For this review, take the finished solid that the model builds, in its own axes (mm). Give positions to 0.01 mm unless a question says otherwise; leave off trailing zeros. Order: outer loops, then holes, each group sorted by start corner. A loop starts at its lowest first (then second) coordinate and runs counter-clockwise, first axis right, second up. Notation, with made-up numbers: (-16, 60.25) -> (26, 60.25) arc R16 cw to (26, 65.25) -> close; hole circle Ø5 at (-20.75, 37). An arc over 180 degrees is marked (long way). Return JSON: item names as keys, results as strings. Group by question number.
1) Add section C-C (z = 1.95). State how many separate pieces and enclosed holes the cut face has, then the cut area to 3 significant figures.
2) Insertion check: P1, Ø3.5, axis at x = 33.61, y = -5.29, coming from the +Z side; P2, Ø1, axis at x = 5, z = 2, coming from the -Y side. Each pin has a flat end and moves straight along its axis. Give the tip position at first contact, or say it passes through.
3) To check wall thickness, follow line 1 along Y through (x, z) = (13, 2.7); line 2 along Y through (x, z) = (3, 1.8); line 3 along Y through (x, z) = (35.5, 1.9). State the ranges of each line that lie inside material, in increasing order.
4) Add section B-B (x = 33). Give the boundary of the cut face in (y, z).
5) Add section D-D (y = 0). Give the boundary of the cut face in (x, z), then the cut area to 3 significant figures.
6) The part is to be moulded in two halves that separate along Y. For faces 1 (the face through (35.094, 10.903, 1.479)), 2 (the face through (-11.237, -34.76, 1.479)), 3 (the face through (-22.86, -10.54, 1.48)), 4 (the face through (19.305, 12.095, 1.479)), say which applies: released by +Y, released by -Y, zero draft, split by the parting line, or undercut.
7) Add section A-A (y = -32). Give the boundary of the cut face in (x, z), then the cut area to 3 significant figures.
from build123d import *

# Parameters (mm, degrees)
SKETCH8_R           = 2.75
SKETCH8_R_2         = 5.3467
BOSS_EXTRUDE1_DEPTH = 3


with BuildPart() as part:
    # Sketch8 → Boss-Extrude1 (new body)
    with BuildSketch(Plane.XY):
        with BuildLine():
            Line((-22.998435926, -22.998435926), (0.859030886, -46.855902739))
            Line((0.859030886, -46.855902739), (46.855902739, -0.859030886))
            Line((46.855902739, -0.859030886), (22.998435926, 22.998435926))
            ThreePointArc((22.998435926, 22.998435926), (10.677524528, 22.998435926), (10.677524528, 10.677524528))
            Line((10.677524528, 10.677524528), (10.668544272, 10.668544272))
            ThreePointArc((10.668544272, 10.668544272), (10.668544272, -10.668544272), (-10.668544272, -10.668544272))
            Line((-10.668544272, -10.668544272), (-10.677524528, -10.677524528))
            ThreePointArc((-10.677524528, -10.677524528), (-22.998435926, -10.677524528), (-22.998435926, -22.998435926))
        make_face()
        with Locations((33.610182952, -5.29098063)):
            Circle(SKETCH8_R, mode=Mode.SUBTRACT)
        with Locations((16.837980227, 16.837980227)):
            Circle(SKETCH8_R_2, mode=Mode.SUBTRACT)
        with Locations((-16.837980227, -16.837980227)):
            Circle(SKETCH8_R_2, mode=Mode.SUBTRACT)
        with Locations((5.325911705, -33.575251877)):
            Circle(SKETCH8_R, mode=Mode.SUBTRACT)
    extrude(amount=BOSS_EXTRUDE1_DEPTH)


solid = part.part
Evaluation:
{
 "1": {"separate pieces": "1", "enclosed holes": "4", "area": "1,850 mm^2"},
 "2": {"P1": "through", "P2": "y = -43.21"},
 "3": {"line 1": "-34.71 to -7.66, 7.66 to 13.12, 20.56 to 24.66", "line 2": "-44.71 to -35.04, -32.11 to -14.79", "line 3": "-12.21 to -7.29, -3.29 to 10.5"},
 "4": {"outline": "(-14.71, 0) -> (-7.97, 0) -> (-7.97, 3) -> (-14.71, 3) -> close; (-2.61, 0) -> (13, 0) -> (13, 3) -> (-2.61, 3) -> close"},
 "5": {"outline": "(15.09, 0) -> (46, 0) -> (46, 3) -> (15.09, 3) -> close", "area": "92.7 mm^2"},
 "6": {"face 1": "released by +Y", "face 2": "released by -Y", "face 3": "split by the parting line", "face 4": "undercut"},
 "7": {"outline": "(-14, 0) -> (3.07, 0) -> (3.07, 3) -> (-14, 3) -> close; (7.58, 0) -> (15.71, 0) -> (15.71, 3) -> (7.58, 3) -> close", "area": "75.6 mm^2"}
}
